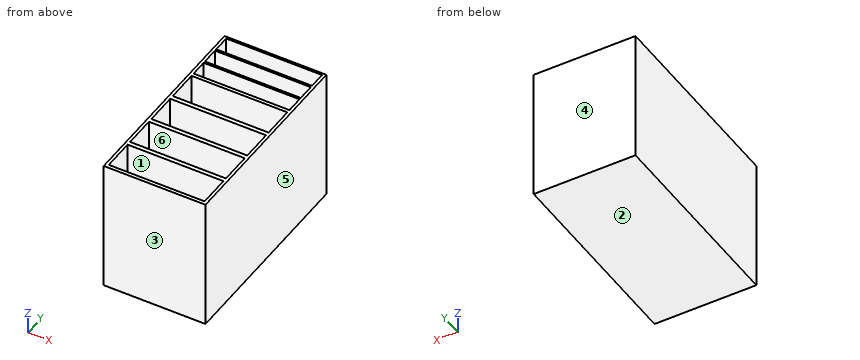
```python
from build123d import *

# Parameters (mm, degrees)
SKETCH1_W           = 72.5
SKETCH1_H           = 95
BOSS_EXTRUDE1_DEPTH = 104.5
SKETCH2_W           = 68.25
SKETCH2_H           = 22.5
CUT_EXTRUDE1_DEPTH  = 90
SKETCH3_W           = 72.5
SKETCH3_H           = 95
BOSS_EXTRUDE2_DEPTH = 175.5
SKETCH4_W           = 68.25
SKETCH4_H           = 12
CUT_EXTRUDE3_DEPTH  = 90
SPLIT1_START        = -36.25
SPLIT1_OUTLINE_W    = 135.5
SPLIT1_OUTLINE_H    = 95
SPLIT1_DEPTH        = 72.5


# Read off the part's stored shape, not the designer's step: Split1
with BuildPart() as part:
    # Sketch1 → Boss-Extrude1 (new body)
    with BuildSketch(Plane(origin=(0, 0, 0), x_dir=(1, 0, 0), z_dir=(0, 1, 0))):
        Rectangle(SKETCH1_W, SKETCH1_H)
    extrude(amount=BOSS_EXTRUDE1_DEPTH)

    # Sketch2 → Cut-Extrude1 (cut)
    with BuildSketch(Plane.XY.offset(47.5)):
        with Locations((0, 13.75)):
            Rectangle(SKETCH2_W, SKETCH2_H)
        with Locations((0, 39.25)):
            Rectangle(SKETCH2_W, SKETCH2_H)
        with Locations((0, 64.75)):
            Rectangle(SKETCH2_W, SKETCH2_H)
        with Locations((0, 90.25)):
            Rectangle(SKETCH2_W, SKETCH2_H)
    extrude(amount=-CUT_EXTRUDE1_DEPTH, mode=Mode.SUBTRACT)

    # Sketch3 → Boss-Extrude2 (add)
    with BuildSketch(Plane(origin=(0, 104.5, 0), x_dir=(1, 0, 0), z_dir=(0, 1, 0))):
        Rectangle(SKETCH3_W, SKETCH3_H)
    extrude(amount=BOSS_EXTRUDE2_DEPTH)

    # Sketch4 → Cut-Extrude3 (cut)
    with BuildSketch(Plane.XY.offset(47.5)):
        with Locations((0, 110)):
            Rectangle(SKETCH4_W, SKETCH4_H)
        with Locations((0, 123.5)):
            Rectangle(SKETCH4_W, SKETCH4_H)
        with Locations((0, 137)):
            Rectangle(SKETCH4_W, SKETCH4_H)
        with Locations((0, 150.5)):
            Rectangle(SKETCH4_W, SKETCH4_H)
        with Locations((0, 164)):
            Rectangle(SKETCH4_W, SKETCH4_H)
        with Locations((0, 177.5)):
            Rectangle(SKETCH4_W, SKETCH4_H)
        with Locations((0, 191)):
            Rectangle(SKETCH4_W, SKETCH4_H)
        with Locations((0, 204.5)):
            Rectangle(SKETCH4_W, SKETCH4_H)
        with Locations((0, 218)):
            Rectangle(SKETCH4_W, SKETCH4_H)
        with Locations((0, 231.5)):
            Rectangle(SKETCH4_W, SKETCH4_H)
        with Locations((0, 245)):
            Rectangle(SKETCH4_W, SKETCH4_H)
        with Locations((0, 258.5)):
            Rectangle(SKETCH4_W, SKETCH4_H)
        with Locations((0, 272)):
            Rectangle(SKETCH4_W, SKETCH4_H)
    extrude(amount=-CUT_EXTRUDE3_DEPTH, mode=Mode.SUBTRACT)

    # Split1 outline → Split1 (cut)
    with BuildSketch(Plane.YZ.offset(SPLIT1_START)):
        with Locations((212.25, 0)):
            Rectangle(SPLIT1_OUTLINE_W, SPLIT1_OUTLINE_H)
    extrude(amount=SPLIT1_DEPTH, mode=Mode.SUBTRACT)


solid = part.part
```
The listing builds one solid part. Answer for the finished solid, in the listing's coordinates (mm). Face numbers are marked on the shaded views. A direction names the side the tool comes from. Coordinates: 2 decimals unless noted, no trailing zeros. Order: outer loops, then holes, each group sorted by start corner. A loop starts at its lowest first (then second) coordinate and runs counter-clockwise, first axis right, second up. Notation, with made-up numbers: M -12,79.25 L -5,79.25 A30 ccw -5,113.25 Z; hole C -26,37 d11. An arc over 180 degrees is marked long. Answer as a JSON object with one key per item and string values. Group by question number.
1. Straight lines are drawn through the part: line 1 (X direction, y = 41, z = 39) (3 decimals); line 2 (Z direction, x = -21, y = 36.5). For each, find the intervals that lie inside material, in ascending order.
2. A tool of negligible diameter and unlimited length cuts with its end or side. For the marked faces 1 and 2, from which of +Z, -Z, +X, -X, +Y, -Y can it reach the whole face along a straight path? Write none if from no direction.
3. A flat-ended cylindrical pin translates along its axis: P1, Ø11, axis at x = -10.5, y = 10, coming from the +Z side. Find the tip coordinate at first contact, or state that the pin passes through.
4. Section C-C on y = 96 is taken. Write down the section's boundary in (x, z) (3 decimals).
5. Determine the mould class of the marked faces 3, 4, 5 and 6 for opening direction Y: released by +Y, released by -Y, zero draft, split by the parting line, or undercut.
6. Section A-A on z = -12 is taken. State how many separate pieces and enclosed holes the cut face has, then the cut area to 3 significant figures.
Values follow:
{
 "1": {"line 1": "-36.25 to -34.125, 34.125 to 36.25", "line 2": "-47.5 to -42.5"},
 "2": {"face 1": "+Z", "face 2": "-Z, +X, -X, +Y, -Y"},
 "3": {"P1": "z = -42.5"},
 "4": {"outline": "M -36.25,-47.5 L 36.25,-47.5 L 36.25,47.5 L 34.125,47.5 L 34.125,-42.5 L -34.125,-42.5 L -34.125,47.5 L -36.25,47.5 Z"},
 "5": {"face 3": "released by -Y", "face 4": "released by +Y", "face 5": "zero draft", "face 6": "undercut"},
 "6": {"separate pieces": "1", "enclosed holes": "7", "area": "1,880 mm2"}
}
